from build123d import *

# Parameters (mm, degrees)
SKETCH1_W           = 70
SKETCH1_H           = 30
SKETCH1_R           = 1.55
BOSS_EXTRUDE1_DEPTH = 17
SKETCH2_R           = 1.55
CUT_EXTRUDE1_DEPTH  = 15


with BuildPart() as part:
    # Sketch1 → Boss-Extrude1 (new body)
    with BuildSketch(Plane.XY):
        Rectangle(SKETCH1_W, SKETCH1_H)
        with Locations((-32, 12)):
            Circle(SKETCH1_R, mode=Mode.SUBTRACT)
        with Locations((32, 12)):
            Circle(SKETCH1_R, mode=Mode.SUBTRACT)
        with Locations((32, -12)):
            Circle(SKETCH1_R, mode=Mode.SUBTRACT)
        with Locations((-32, -12)):
            Circle(SKETCH1_R, mode=Mode.SUBTRACT)
    extrude(amount=BOSS_EXTRUDE1_DEPTH)

    # Sketch2 → Cut-Extrude1 (cut)
    with BuildSketch(Plane.XY.offset(17)):
        with BuildLine():
            Line((-35, 15), (-35, 5))
            ThreePointArc((-35, 5), (-27.928932188, 7.928932188), (-25, 15))
            Line((-25, 15), (-35, 15))
        make_face()
        with Locations((-32, 12)):
            Circle(SKETCH2_R, mode=Mode.SUBTRACT)
        with BuildLine():
            Line((35, 15), (25, 15))
            ThreePointArc((25, 15), (27.928932188, 7.928932188), (35, 5))
            Line((35, 5), (35, 15))
        make_face()
        with Locations((32, 12)):
            Circle(SKETCH2_R, mode=Mode.SUBTRACT)
        with BuildLine():
            ThreePointArc((35, -5), (27.928932188, -7.928932188), (25, -15))
            Line((25, -15), (35, -15))
            Line((35, -15), (35, -5))
        make_face()
        with Locations((32, -12)):
            Circle(SKETCH2_R, mode=Mode.SUBTRACT)
        with BuildLine():
            ThreePointArc((-25, -15), (-27.928932188, -7.928932188), (-35, -5))
            Line((-35, -5), (-35, -15))
            Line((-35, -15), (-25, -15))
        make_face()
        with Locations((-32, -12)):
            Circle(SKETCH2_R, mode=Mode.SUBTRACT)
    extrude(amount=-CUT_EXTRUDE1_DEPTH, mode=Mode.SUBTRACT)


solid = part.part
Can you work these out from the model? Positions are in its coordinate system, mm. A direction names the side the tool comes from. Give positions to 0.01 mm unless a question says otherwise; leave off trailing zeros. Loops run counter-clockwise (first coordinate to the right, second up) from the corner with the lowest first, then second, coordinate; pieces in that order, holes last. Notation, with made-up numbers: (-11.5, 2.5) - (23.5, 2.5) arc R16 ccw to (23.5, 31.5) - close; hole circle Ø11 at (73, 19.5). An arc over 180 degrees is marked (long way). One line per item, written item: value.
(1) If we section it at A-A, the plane x = -27: List the corners of the cut face in (y, z) for me, plus the area to 3 significant figures.
Verdict:
outline: (-15, 0) - (15, 0) - (15, 2) - (9, 2) - (9, 17) - (-9, 17) - (-9, 2) - (-15, 2) - close
area: 330 mm^2
(2) On a 3-axis mill with a long thin cutter (end or side, diameter ignored), from which of +Z, -Z, +X, -X, +Y, -Y can I reach the whole of each face in a straight line? I mean faces 5 (the face through (0, 15, 8)), 6 (the face through (-30, 11, 2)), 7 (the face through (30, 11, 2)), 8 (the face through (28.01, -7.85, 9.6)), 9 (the face through (-31, -10, 2)). Say none if no direction works.
Verdict:
face 5: +Z, -Z, +X, -X, +Y
face 6: +Z, -X, +Y
face 7: +Z, +X, +Y
face 8: +Z, +X, -Y
face 9: +Z, -X, -Y
(3) I need wall thicknesses on line 1 along Y through (x, z) = (32, 0.85); line 2 along X through (y, z) = (8.25, 3); line 3 along X through (y, z) = (-6.25, 14.5). Which ranges of each line are inside material? Lowest first, please.
Verdict:
line 1: -15 to -13.55, -10.45 to 10.45, 13.55 to 15
line 2: -27.62 to 27.62
line 3: -30.16 to 30.16
(4) If we section it at B-B, the plane z = 10: List the corners of the cut face in (x, y) for me.
Verdict:
outline: (-35, -5) arc R10 cw to (-25, -15) - (25, -15) arc R10 cw to (35, -5) - (35, 5) arc R10 cw to (25, 15) - (-25, 15) arc R10 cw to (-35, 5) - close
(5) If we mould it in two halves opening along X, with no side actions, what happens to faces 1 (the face through (33.478, -11.534, 0.986)), 2 (the face through (30, -11, 2)), 3 (the face through (-30.568, 11.406, 0.986)), 4 (the face through (27.85, 8.01, 9.6))? For each: released by +X, released by -X, zero draft, split by the parting line, or undercut.
Verdict:
face 1: undercut
face 2: zero draft
face 3: undercut
face 4: released by +X
(6) I'm going to push flat-ended pins straight in: pin 1 (1.9 mm diameter, centred on x = 32, y = 12, fed in from +Z); pin 2 (3.5 mm diameter, centred on x = -32, y = -12, fed in from +Z); pin 3 (10 mm diameter, centred on y = -11.5, z = 14.5, fed in from -X). Where does each tip first touch, or does it pass through?
Verdict:
pin 1: through
pin 2: z = 2
pin 3: x = -29.73
